Geometry: final body of the model. Coordinates: model frame, mm. Face numbers are marked on the shaded views. A direction names the side the tool comes from. Coordinates: 2 decimals unless noted, no trailing zeros. Order: outer loops, then holes, each group sorted by start corner. A loop starts at its lowest first (then second) coordinate and runs counter-clockwise, first axis right, second up. Notation, with made-up numbers: (-31.75, 53.5) -> (-24.75, 53.5) arc R26 ccw to (-24.75, 75.5) -> close; hole circle Ø1 at (-3, 49). An arc over 180 degrees is marked (long way). Use CSV: the item, a comma, the result in double quotes. Start each with the question number.
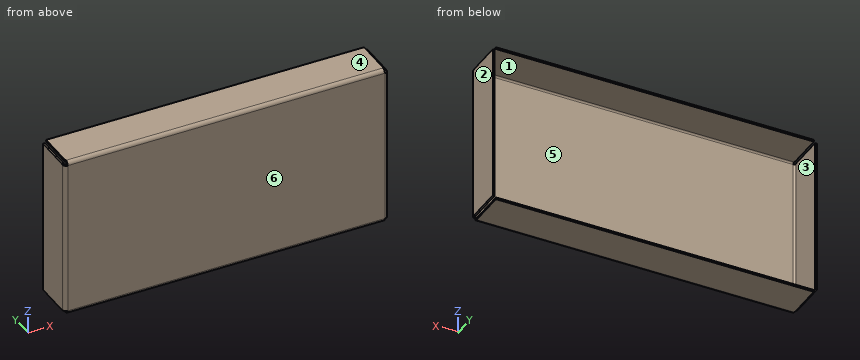
from build123d import *

# Parameters (mm, degrees)
SKETCH1_W              = 152.4
SKETCH1_H              = 76.2
BOSS_EXTRUDE1_DEPTH    = 19.05
CONVERT_SOLID1_START   = -74.5236
CONVERT_SOLID1_DEPTH   = 72.8472
CONVERT_SOLID1_START_2 = -77
CONVERT_SOLID1_2_DEPTH = 2.273736392
CONVERT_SOLID1_START_3 = -1.473736392
CONVERT_SOLID1_3_DEPTH = 2.473736392
CONVERT_SOLID1_START_4 = -74.726263608
CONVERT_SOLID1_4_DEPTH = 73.252527216
CONVERT_SOLID1_5_DEPTH = 0.202663608
CONVERT_SOLID1_START_5 = -1.6764
CONVERT_SOLID1_6_DEPTH = 0.202663608
CONVERT_SOLID1_START_6 = 1.473736392
CONVERT_SOLID1_7_DEPTH = 149.452527216


with BuildPart() as part:
    # Sketch1 → Boss-Extrude1 (new body)
    with BuildSketch(Plane(origin=(0, 0, 0), x_dir=(1, 0, 0), z_dir=(0, 1, 0))):
        with Locations((76.2, 38.1)):
            Rectangle(SKETCH1_W, SKETCH1_H)
    extrude(amount=BOSS_EXTRUDE1_DEPTH)

    # Convert-Solid1: read off the stored shape, not the designer's step
    # Convert-Solid1 outline → Convert-Solid1 (cut)
    with BuildSketch(Plane.XY.offset(CONVERT_SOLID1_START)):
        with BuildLine():
            Line((151.511, 19.05), (0.889, 19.05))
            Line((0.889, 19.05), (0.889, 1.6764))
            ThreePointArc((0.889, 1.6764), (1.11962412, 1.11962412), (1.6764, 0.889))
            Line((1.6764, 0.889), (150.7236, 0.889))
            ThreePointArc((150.7236, 0.889), (151.28037588, 1.11962412), (151.511, 1.6764))
            Line((151.511, 1.6764), (151.511, 19.05))
        make_face()
        with BuildLine():
            ThreePointArc((152.4, 1.6764), (151.908993808, 0.491006192), (150.7236, 0))
            Line((150.7236, 0), (152.4, 0))
            Line((152.4, 0), (152.4, 1.6764))
        make_face()
        with BuildLine():
            Line((0, 0), (1.6764, 0))
            ThreePointArc((1.6764, 0), (0.491006192, 0.491006192), (0, 1.6764))
            Line((0, 1.6764), (0, 0))
        make_face()
    extrude(amount=CONVERT_SOLID1_DEPTH, mode=Mode.SUBTRACT)

    # Convert-Solid1 2 outline → Convert-Solid1 2 (cut)
    with BuildSketch(Plane.XY.offset(CONVERT_SOLID1_START_2)):
        Polygon((150.926263608, 2.11106664), (150.7236, 2.11106664), (150.7236, 0), (152.4, 0), (152.4, 19.05), (150.926263608, 19.05), align=None)
        Polygon((1.473736392, 19.05), (0, 19.05), (0, 0), (1.6764, 0), (1.6764, 2.11106664), (1.473736392, 2.11106664), align=None)
    extrude(amount=CONVERT_SOLID1_2_DEPTH, mode=Mode.SUBTRACT)

    # Convert-Solid1 3 outline → Convert-Solid1 3 (cut)
    with BuildSketch(Plane.XY.offset(CONVERT_SOLID1_START_3)):
        Polygon((150.926263608, 2.11106664), (150.7236, 2.11106664), (150.7236, 0), (152.4, 0), (152.4, 19.05), (150.926263608, 19.05), align=None)
        Polygon((1.473736392, 19.05), (0, 19.05), (0, 0), (1.6764, 0), (1.6764, 2.11106664), (1.473736392, 2.11106664), align=None)
    extrude(amount=CONVERT_SOLID1_3_DEPTH, mode=Mode.SUBTRACT)

    # Convert-Solid1 4 outline → Convert-Solid1 4 (cut)
    with BuildSketch(Plane.XY.offset(CONVERT_SOLID1_START_4)):
        with BuildLine():
            Line((150.926263608, 2.11106664), (150.7236, 2.11106664))
            Line((150.7236, 2.11106664), (150.7236, 0.889))
            ThreePointArc((150.7236, 0.889), (151.28037588, 1.11962412), (151.511, 1.6764))
            Line((151.511, 1.6764), (151.511, 19.05))
            Line((151.511, 19.05), (150.926263608, 19.05))
            Line((150.926263608, 19.05), (150.926263608, 2.11106664))
        make_face()
        with BuildLine():
            ThreePointArc((152.4, 1.6764), (151.908993808, 0.491006192), (150.7236, 0))
            Line((150.7236, 0), (152.4, 0))
            Line((152.4, 0), (152.4, 1.6764))
        make_face()
        with BuildLine():
            ThreePointArc((0.889, 1.6764), (1.11962412, 1.11962412), (1.6764, 0.889))
            Line((1.6764, 0.889), (1.6764, 2.11106664))
            Line((1.6764, 2.11106664), (1.473736392, 2.11106664))
            Line((1.473736392, 2.11106664), (1.473736392, 19.05))
            Line((1.473736392, 19.05), (0.889, 19.05))
            Line((0.889, 19.05), (0.889, 1.6764))
        make_face()
        with BuildLine():
            Line((0, 0), (1.6764, 0))
            ThreePointArc((1.6764, 0), (0.491006192, 0.491006192), (0, 1.6764))
            Line((0, 1.6764), (0, 0))
        make_face()
    extrude(amount=CONVERT_SOLID1_4_DEPTH, mode=Mode.SUBTRACT)

    # Convert-Solid1 5 outline → Convert-Solid1 5 (cut)
    with BuildSketch(Plane.XY.offset(CONVERT_SOLID1_START_4)):
        with BuildLine():
            ThreePointArc((151.511, 1.6764), (151.28037588, 1.11962412), (150.7236, 0.889))
            Line((150.7236, 0.889), (150.7236, 0))
            ThreePointArc((150.7236, 0), (151.908993808, 0.491006192), (152.4, 1.6764))
            Line((152.4, 1.6764), (152.4, 2.11106664))
            Line((152.4, 2.11106664), (151.511, 2.11106664))
            Line((151.511, 2.11106664), (151.511, 1.6764))
        make_face()
        with BuildLine():
            Line((1.6764, 0), (1.6764, 0.889))
            ThreePointArc((1.6764, 0.889), (1.11962412, 1.11962412), (0.889, 1.6764))
            Line((0.889, 1.6764), (0.889, 2.11106664))
            Line((0.889, 2.11106664), (0, 2.11106664))
            Line((0, 2.11106664), (0, 1.6764))
            ThreePointArc((0, 1.6764), (0.491006192, 0.491006192), (1.6764, 0))
        make_face()
    extrude(amount=CONVERT_SOLID1_5_DEPTH, mode=Mode.SUBTRACT)

    # Convert-Solid1 6 outline → Convert-Solid1 6 (cut)
    with BuildSketch(Plane.XY.offset(CONVERT_SOLID1_START_5)):
        with BuildLine():
            ThreePointArc((151.511, 1.6764), (151.28037588, 1.11962412), (150.7236, 0.889))
            Line((150.7236, 0.889), (150.7236, 0))
            ThreePointArc((150.7236, 0), (151.908993808, 0.491006192), (152.4, 1.6764))
            Line((152.4, 1.6764), (152.4, 2.11106664))
            Line((152.4, 2.11106664), (151.511, 2.11106664))
            Line((151.511, 2.11106664), (151.511, 1.6764))
        make_face()
        with BuildLine():
            Line((1.6764, 0), (1.6764, 0.889))
            ThreePointArc((1.6764, 0.889), (1.11962412, 1.11962412), (0.889, 1.6764))
            Line((0.889, 1.6764), (0.889, 2.11106664))
            Line((0.889, 2.11106664), (0, 2.11106664))
            Line((0, 2.11106664), (0, 1.6764))
            ThreePointArc((0, 1.6764), (0.491006192, 0.491006192), (1.6764, 0))
        make_face()
    extrude(amount=CONVERT_SOLID1_6_DEPTH, mode=Mode.SUBTRACT)

    # Convert-Solid1 7 outline → Convert-Solid1 7 (cut)
    with BuildSketch(Plane.YZ.offset(CONVERT_SOLID1_START_6)):
        with BuildLine():
            Line((0, 0), (0, -1.6764))
            ThreePointArc((0, -1.6764), (0.491006192, -0.491006192), (1.6764, 0))
            Line((1.6764, 0), (0, 0))
        make_face()
        with BuildLine():
            ThreePointArc((1.6764, -76.2), (0.491006192, -75.708993808), (0, -74.5236))
            Line((0, -74.5236), (0, -76.2))
            Line((0, -76.2), (1.6764, -76.2))
        make_face()
        with BuildLine():
            Line((19.05, -74.5236), (0.889, -74.5236))
            ThreePointArc((0.889, -74.5236), (1.11962412, -75.08037588), (1.6764, -75.311))
            Line((1.6764, -75.311), (19.05, -75.311))
            Line((19.05, -75.311), (19.05, -74.5236))
        make_face()
        with BuildLine():
            Line((0.889, -1.6764), (19.05, -1.6764))
            Line((19.05, -1.6764), (19.05, -0.889))
            Line((19.05, -0.889), (1.6764, -0.889))
            ThreePointArc((1.6764, -0.889), (1.11962412, -1.11962412), (0.889, -1.6764))
        make_face()
    extrude(amount=CONVERT_SOLID1_7_DEPTH, mode=Mode.SUBTRACT)


solid = part.part
(1) Line query: line 1 (X direction, y = 12, z = -4); line 2 (Z direction, x = 90.5, y = 17.25); line 3 (Y direction, x = 56, z = -32). Output: solid intervals per line, ascending. Write a range as from..to.
(2) Section C-C (x = 76.5). Return loops of the section in (y, z).
(3) Mould query, pull axis Z, two halves, no side actions, for the marked faces 4, 5 and 6. Classes: pulls with the +Z half, pulls with the -Z half, needs draft (parallel to the pull), parting line crosses it, or undercut.
(4) First-contact query: pin 1 (0.8 mm diameter, centred on y = 1, z = -1, fed in from -X); pin 2 (6 mm diameter, centred on x = 39, z = -9.5, fed in from +Y); pin 3 (8.5 mm diameter, centred on y = 13, z = -22, fed in from -X); pin 4 (0.5 mm diameter, centred on x = 0.5, y = 0.5, fed in from -Z). Flat tips, straight axial feed; report the tip coordinate or a pass-through.
(5) Section B-B (z = -6). Return loops of the section in (x, y).
(6) Section A-A (y = 17.5). Return loops of the section in (x, z), then the cut area to 3 significant figures.
(7) Access query for the marked faces 1, 2 and 3. Directions: +Z, -Z, +X, -X, +Y, -Y. A direction counts if a zero-diameter tool reaches every point of the face in a straight line with its end or side. Return the directions, or none.
Check sheet entries:
1,line 1,"x = 0..0.89, 151.51..152.4"
1,line 2,"z = -76.2..-75.31, -0.89..0"
1,line 3,"y = 0..0.89"
2,outline,"(0, -74.52) arc R1.68 ccw to (1.68, -76.2) -> (19.05, -76.2) -> (19.05, -75.31) -> (1.68, -75.31) arc R0.79 cw to (0.89, -74.52) -> (0.89, -1.68) arc R0.79 cw to (1.68, -0.89) -> (19.05, -0.89) -> (19.05, 0) -> (1.68, 0) arc R1.68 ccw to (0, -1.68) -> close"
3,face 4,"pulls with the +Z half"
3,face 5,"undercut"
3,face 6,"needs draft"
4,pin 1,"stops at x = 1.68"
4,pin 2,"stops at y = 0.89"
4,pin 3,"stops at x = 0"
4,pin 4,"stops at z = -74.52"
5,outline,"(0, 1.68) arc R1.68 ccw to (1.68, 0) -> (150.72, 0) arc R1.68 ccw to (152.4, 1.68) -> (152.4, 19.05) -> (151.51, 19.05) -> (151.51, 1.68) arc R0.79 cw to (150.72, 0.89) -> (1.68, 0.89) arc R0.79 cw to (0.89, 1.68) -> (0.89, 19.05) -> (0, 19.05) -> close"
6,outline,"(0, -74.73) -> (0.89, -74.73) -> (0.89, -1.47) -> (0, -1.47) -> close; (1.47, -76.2) -> (150.93, -76.2) -> (150.93, -75.31) -> (1.47, -75.31) -> close; (1.47, -0.89) -> (150.93, -0.89) -> (150.93, 0) -> (1.47, 0) -> close; (151.51, -74.73) -> (152.4, -74.73) -> (152.4, -1.47) -> (151.51, -1.47) -> close"
6,area,"396 mm^2"
7,face 1,"+X, -X, +Y"
7,face 2,"+Z, -Z, +X, +Y, -Y"
7,face 3,"+Z, -Z, +Y"
